Could you check a few things on this drawing? It's one solid part, dimensions in mm from its lowest x, y, z. Give positions to 0.01 mm unless a question says otherwise; leave off trailing zeros. Loops run counter-clockwise (first coordinate to the right, second up) from the corner with the lowest first, then second, coordinate; pieces in that order, holes last. Notation, with made-up numbers: M -32.5,80.25 L -22.5,80.25 A26 cw -22.5,103.25 Z; hole C 8,19 d10. An arc over 180 degrees is marked long. Answer in a Markdown table with one row per item. Add a question column.
1. I need wall thicknesses on line 1 along X through (y, z) = (1.05, 58.5) (1 decimal); line 2 along X through (y, z) = (0.1, 80); line 3 along Z through (x, y) = (37.5, 1.9). Which ranges of each line are inside material? Lowest first, please. Write a range as from..to.
2. If we section it at B-B on y = 0.95: Count the separate pieces of the cut face and the enclosed holes in it, then the cut area to 3 significant figures.
3. If we section it at D-D on z = 13: List the corners of the cut face in (x, y) for me, then the cut area to 3 significant figures.
4. If we section it at A-A on z = 36: List the corners of the cut face in (x, y) for me.
5. I'm going to push a flat-ended pin straight in: pin 1 Ø2 at (x, z) = (79.5, 99) entering from -Y. Where does the tip first touch, or does it pass through?
6. If we section it at C-C on x = 74: List the corners of the cut face in (y, z) for me.
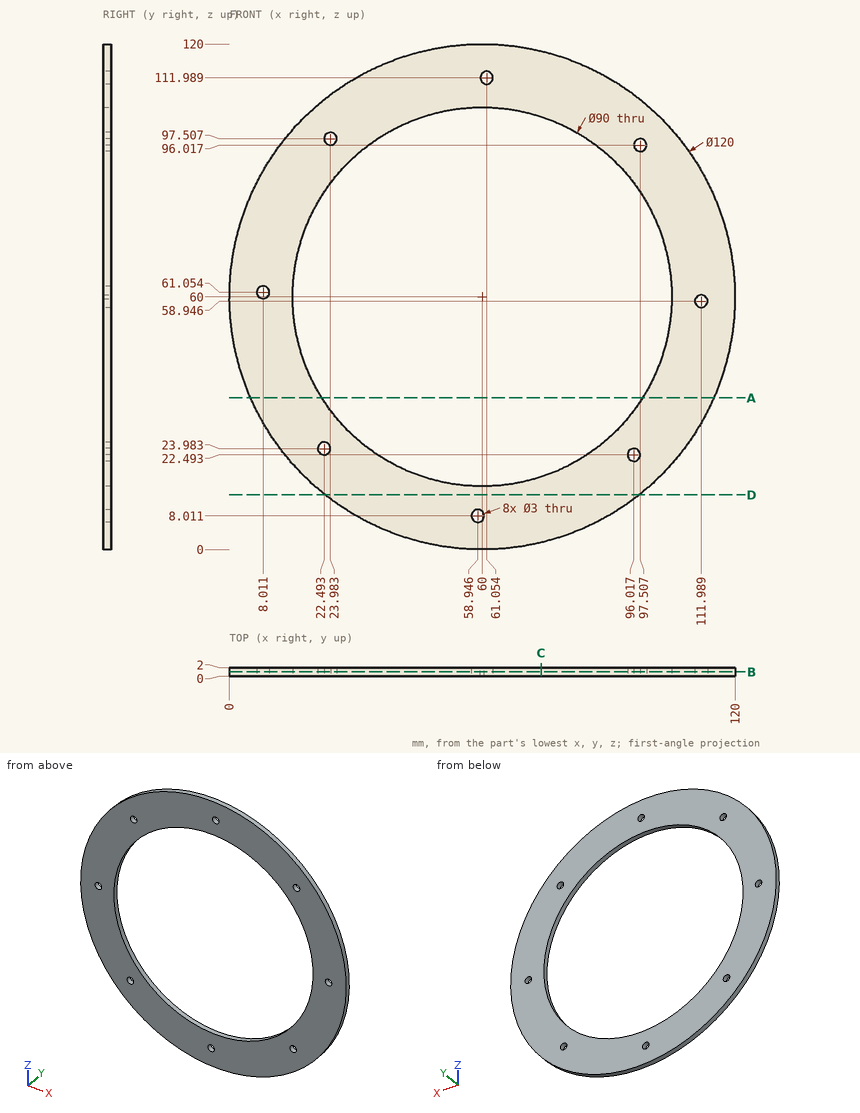
Results:
| question | item | result |
|---|---|---|
| 1 | line 1 | 0..15, 105..110.6, 113.4..120 |
| 1 | line 2 | 3.43..19.69, 100.31..116.57 |
| 1 | line 3 | 4.38..21.03, 98.97..115.62 |
| 2 | separate pieces | 1 |
| 2 | enclosed holes | 9 |
| 2 | area | 4,890 mm2 |
| 3 | outline | M 22.7,0 L 97.3,0 L 97.3,2 L 22.7,2 Z |
| 3 | area | 149 mm2 |
| 4 | outline | M 5.01,0 L 21.93,0 L 21.93,2 L 5.01,2 Z; M 98.07,0 L 114.99,0 L 114.99,2 L 98.07,2 Z |
| 5 | pin 1 | through |
| 6 | outline | M 0,1.66 L 2,1.66 L 2,17.23 L 0,17.23 Z; M 0,102.77 L 2,102.77 L 2,118.34 L 0,118.34 Z |
